Design review of the part built by this model. Coordinates are the model's own, in mm. A direction names the side the tool comes from. Round coordinates to 2 decimals unless told otherwise and drop trailing zeros. Order: outer loops, then holes, each group sorted by start corner. A loop starts at its lowest first (then second) coordinate and runs counter-clockwise, first axis right, second up. Notation, with made-up numbers: M -28.75,61 L -19.75,61 A23 cw -19.75,75 Z; hole C 0.25,-13.75 d7. An arc over 180 degrees is marked long. Use a Markdown table: item, result. Add a question column.
(1) Take a section at A-A (x = 62.5). Write out the cut boundary in (y, z).
(2) To check wall thickness, follow probe 1 along Y at (x, z) = (13, 2.75); probe 2 along X at (y, z) = (-19, 0.6); probe 3 along Y at (x, z) = (-21, 1). State the ranges of each line that lie inside material, in increasing order. Write a range as from..to.
(3) Machinability: for faces 1 (the face through (15, 18.806, 2)), 2 (the face through (45, -35, 2)), which of the approach directions +Z, -Z, +X, -X, +Y, -Y give a long, thin tool a straight path to every point of the face, cutting with its end or side? Answer none if there is none.
(4) Take a section at B-B (x = -6). Write out the cut boundary in (y, z), then the cut area to 3 significant figures.
(5) For pin 1 (1.5 mm diameter, centred on x = 52.5, z = 2, fed in from -Y); pin 2 (1.5 mm diameter, centred on x = -50.5, z = 2.5, fed in from +Y); pin 3 (2.5 mm diameter, centred on x = 10.02, y = -26.43, fed in from +Z), all flat-tipped, find the tip position at first contact; note any pin that passes through.
(6) The part is to be moulded in two halves that separate along Y. For faces 3 (the face through (-80, 0, 2)), 4 (the face through (-62, -27.5, 2)), 5 (the face through (-20, 31.533, 2)), say which applies: released by +Y, released by -Y, zero draft, split by the parting line, or undercut.
(7) Take a section at C-C (z = 1). Count the separate pieces of the cut face and the enclosed holes in it, then the cut area to 3 significant figures.
Autodesk Inventor part; units mm, degrees
ref_plane "YZ Plane" through (0, 0, 0) normal (1, 0, 0) x (0, 1, 0)
ref_plane "XZ Plane" through (0, 0, 0) normal (0, 1, 0) x (-1, 0, 0)
ref_plane "XY Plane" through (0, 0, 0) normal (0, 0, 1) x (1, 0, 0)
sketch "草图1" plane through (0, 0, 0) normal (0, 0, 1) x (1, 0, 0)
  line L0 (45, -42.5) -> (-45, -42.5)
  line L1 (-80, -27.5) -> (-80, 27.5)
  line L2 (-45, 42.5) -> (45, 42.5)
  line L3 (80, 27.5) -> (80, -27.5)
  line L4 (80, -42.5) -> (-80, 42.5) construction
  line L5 (-80, -42.5) -> (80, 42.5) construction
  line L6 (-80, -42.5) -> (-45, -42.5) construction
  line L7 (-45, -42.5) -> (-45, -27.5)
  line L8 (-45, -27.5) -> (-80, -27.5)
  line L9 (-80, -27.5) -> (-80, -42.5) construction
  line L10 (0, 0) -> (-55.8676, 0) construction
  line L11 (0, 0) -> (0, 33.8788) construction
  line L12 (-45, 42.5) -> (-45, 27.5)
  line L13 (-45, 27.5) -> (-80, 27.5)
  line L14 (45, -42.5) -> (45, -27.5)
  line L15 (45, -27.5) -> (80, -27.5)
  line L16 (45, 27.5) -> (80, 27.5)
  line L17 (45, 42.5) -> (45, 27.5)
  line L18 (-39.4263, 5.5352) -> (-42.3668, 0)
  line L19 (-30.1527, 5.5352) -> (-33.0933, 0)
  line L20 (-39.4263, -5.5352) -> (-42.3668, 0)
  line L21 (-30.1527, -5.5352) -> (-33.0933, 0)
  line L22 (-39.4263, 5.5352) -> (-40.4535, 0)
  line L23 (-30.1527, 5.5352) -> (-31.18, 0)
  line L24 (-39.4263, -5.5352) -> (-40.4535, 0)
  line L25 (-30.1527, -5.5352) -> (-31.18, 0)
  line L26 (5.0329, -1.6) -> (-21.3413, -1.6)
  line L27 (-21.3413, 1.6) -> (5.0329, 1.6)
  line L28 (5.0329, 1.6) -> (5.0329, -1.6)
  line L29 (5.0329, -1.6) -> (-21.3413, 1.6) construction
  line L30 (-21.3413, -1.6) -> (5.0329, 1.6) construction
  line L31 (-21.3413, 1.6) -> (-25.0273, 0)
  line L32 (-21.3413, -1.6) -> (-24.8785, 0.0646)
  line L33 (-56.6923, -25.2441) -> (103.3077, 59.7559) construction
  line L34 (28.5415, 15.6059) -> (1.7655, 15.6059)
  line L35 (1.7655, 18.8059) -> (28.5415, 18.8059)
  line L36 (28.5415, 18.8059) -> (28.5415, 15.6059)
  line L37 (1.7655, 18.8059) -> (-1.7578, 17.2389)
  line L38 (1.7655, 15.6059) -> (-1.7197, 17.2559)
  line L39 (1.7655, -18.8059) -> (28.5415, -18.8059)
  line L40 (28.5415, -18.8059) -> (28.5415, -15.6059)
  line L41 (28.5415, -15.6059) -> (1.7655, -15.6059)
  line L42 (1.7655, -15.6059) -> (-1.7197, -17.2559)
  line L43 (1.7655, -18.8059) -> (-1.7578, -17.2389)
  line L44 (-27.9338, 31.5327) -> (-11.0458, 31.5327)
  line L45 (-11.0458, 31.5327) -> (-11.0458, 29.5322)
  line L46 (-11.0458, 29.5322) -> (-27.9338, 29.5322)
  line L47 (-27.9338, 29.5322) -> (-27.9338, 31.5327)
  line L48 (-27.9338, -31.5327) -> (-11.0458, -31.5327)
  line L49 (-11.0458, -31.5327) -> (-11.0458, -29.5322)
  line L50 (-11.0458, -29.5322) -> (-27.9338, -29.5322)
  line L51 (-27.9338, -29.5322) -> (-27.9338, -31.5327)
  line L52 (-21.3413, 1.6) -> (-21.3413, -1.6) construction
  point P0 (-62.5, 19.2523)
  point P1 (-47.5406, 19.2523)
  point P2 (-34.2099, 37.9926)
  point P3 (-16.4356, 37.9926)
  point P4 (-62.5, -19.2523)
  point P5 (-47.5406, -19.2523)
  point P6 (-34.2099, -37.9926)
  point P7 (-16.4356, -37.9926)
  point P8 (0, 37.9926)
  point P9 (62.5, 19.2523)
  point P10 (47.5406, 19.2523)
  point P11 (34.2099, 37.9926)
  point P12 (16.4356, 37.9926)
  point P13 (16.4356, -37.9926)
  point P14 (34.2099, -37.9926)
  point P15 (47.5406, -19.2523)
  point P16 (62.5, -19.2523)
  point P17 (-8.1542, 0)
  point P18 (-27.9338, 21.1189)
  point P19 (-12.8958, 21.1189)
  point P20 (-15.067, 10.9368)
  point P21 (-54.892, 8.4055)
  point P22 (-27.9338, -21.1189)
  point P23 (-12.8958, -21.1189)
  point P24 (-15.067, -10.9368)
  point P25 (-54.892, -8.4055)
  point P26 (54.892, 8.4055)
  point P27 (54.892, -8.4055)
  point P28 (15.067, 10.9368)
  point P29 (15.067, -10.9368)
  point P30 (34.2099, 8.4055)
  point P31 (34.2099, -8.4055)
  point P32 (10.0228, 26.427)
  point P33 (10.0228, -26.427)
  point P34 (-75.9408, -22.7627)
  point P35 (-75.9408, 22.7627)
  point P36 (75.9408, -22.7627)
  point P37 (75.9408, 22.7627)
  point P38 (-75.9408, 0)
  point P39 (75.9408, 0)
  dimension "d2" = 35
  dimension "d3" = 15
  dimension "d5" = 3.2
  dimension "d6" = 85
  dimension "d7" = 160
  dimension "d31" = 3.2
extrude "拉伸1" add sketch "草图1" along normal blind 4
hole "孔1" at (-62.5, 19.2523, 0) at (-47.5406, 19.2523, 0) at (-34.2099, 37.9926, 0) at (-16.4356, 37.9926, 0) at (-16.4356, -37.9926, 0) at (-34.2099, -37.9926, 0) at (-47.5406, -19.2523, 0) at (-62.5, -19.2523, 0) at (0, 37.9926, 0) at (34.2099, 37.9926, 0) at (16.4356, 37.9926, 0) at (47.5406, 19.2523, 0) at (62.5, 19.2523, 0) at (47.5406, -19.2523, 0) at (62.5, -19.2523, 0) at (34.2099, -37.9926, 0) at (16.4356, -37.9926, 0) at (-27.9338, 21.1189, 0) at (-12.8958, 21.1189, 0) at (-15.067, 10.9368, 0) at (-54.892, 8.4055, 0) at (-54.892, -8.4055, 0) at (-15.067, -10.9368, 0) at (-12.8958, -21.1189, 0) at (-27.9338, -21.1189, 0) at (54.892, -8.4055, 0) at (54.892, 8.4055, 0) at (15.067, 10.9368, 0) at (15.067, -10.9368, 0) at (34.2099, 8.4055, 0) at (34.2099, -8.4055, 0) at (10.0228, 26.427, 0) at (10.0228, -26.427, 0) direction (0, 0, 1) diameter 3.2 end through all
hole "孔2" at (-75.9408, -22.7627, 0) at (-75.9408, 22.7627, 0) at (75.9408, -22.7627, 0) at (75.9408, 22.7627, 0) direction (0, 0, 1) diameter 3.2 end through all
hole "孔3" at (-75.9408, 0, 0) at (75.9408, 0, 0) direction (0, 0, 1) diameter 3.2 end through all
properties part number "底盘设计3.0" material "聚碳酸酯，透明"
Verdict:
| question | item | result |
|---|---|---|
| 1 | outline | M -27.5,0 L -20.85,0 L -20.85,4 L -27.5,4 Z; M -17.65,0 L 17.65,0 L 17.65,4 L -17.65,4 Z; M 20.85,0 L 27.5,0 L 27.5,4 L 20.85,4 Z |
| 2 | probe 1 | y = -42.5..-18.81, -15.61..15.61, 18.81..42.5 |
| 2 | probe 2 | x = -80..-64.08, -60.92..-49.12, -45.96..45.96, 49.12..60.92, 64.08..80 |
| 2 | probe 3 | y = -42.5..-31.53, -29.53..-1.6, 1.6..29.53, 31.53..42.5 |
| 3 | face 1 | +Z, -Z |
| 3 | face 2 | +Z, -Z, +X, -Y |
| 4 | outline | M -42.5,0 L -1.6,0 L -1.6,4 L -42.5,4 Z; M 1.6,0 L 42.5,0 L 42.5,4 L 1.6,4 Z |
| 4 | area | 327 mm^2 |
| 5 | pin 1 | stops at y = -27.5 |
| 5 | pin 2 | stops at y = 27.5 |
| 5 | pin 3 | passes through |
| 6 | face 3 | zero draft |
| 6 | face 4 | released by -Y |
| 6 | face 5 | undercut |
| 7 | separate pieces | 1 |
| 7 | enclosed holes | 46 |
| 7 | area | 10,800 mm^2 |
